Here's how the part is built. I have some questions about the finished solid (model axes, mm). Give positions to 0.01 mm unless a question says otherwise; leave off trailing zeros. Loops run counter-clockwise (first coordinate to the right, second up) from the corner with the lowest first, then second, coordinate; pieces in that order, holes last. Notation, with made-up numbers: (29.5, 76) - (60.5, 76) arc R14 ccw to (60.5, 99) - close; hole circle Ø4 at (34.5, -27.5). An arc over 180 degrees is marked (long way). Use a Markdown table: item, result.
from build123d import *

# Parameters (mm, degrees)
BOSS_EXTRUDE2_DEPTH = 0.2
BOSS_EXTRUDE3_DEPTH = 0.2


with BuildPart() as part:
    # Sketch1 → Revolve1 (revolve)
    with BuildSketch(Plane.XY):
        with BuildLine():
            Line((-1.375, 7.8), (1.375, 7.8))
            Line((1.375, 7.8), (1.375, 12.1))
            ThreePointArc((1.375, 12.1), (1.169974747, 12.594974747), (0.675, 12.8))
            Line((0.675, 12.8), (0.625, 12.8))
            Line((0.625, 12.8), (0.625, 13.6))
            ThreePointArc((0.625, 13.6), (0.478553391, 13.953553391), (0.125, 14.1))
            Line((0.125, 14.1), (-1.075, 14.1))
            ThreePointArc((-1.075, 14.1), (-1.287132034, 14.012132034), (-1.375, 13.8))
            Line((-1.375, 13.8), (-1.375, 7.8))
        make_face()
    revolve(axis=Axis((-11.93322357, 7.8, 0), (1, 0, 0)))

    # Sketch3 → Boss-Extrude2 (add)
    with BuildSketch(Plane(origin=(1.375, 0, 0), x_dir=(0, 0, -1), z_dir=(1, 0, 0))):
        Polygon((-2, 8), (-2, -1), (-1.25, -1), (-1.25, 0), (1.25, 0), (1.25, 8), align=None)
    extrude(amount=BOSS_EXTRUDE2_DEPTH)

    # Sketch5 → Boss-Extrude3 (add)
    with BuildSketch(Plane(origin=(-1.375, 0, -1.375), x_dir=(0, 0, -1), z_dir=(1, 0, 0))):
        Polygon((0.625, -1), (0.625, 8), (-2.625, 8), (-2.625, 0), (-0.125, 0), (-0.125, -1), align=None)
    extrude(amount=-BOSS_EXTRUDE3_DEPTH)


solid = part.part
(1) Suppose I cut it at C-C on y = 7.8. Write out the boundary of the cut face in (x, z) (3 decimals).
A:
| item | result |
|---|---|
| outline | (-1.575, -2) - (-1.375, -2) - (-1.375, -6) arc R0.3 ccw to (-1.075, -6.3) - (0.125, -6.3) arc R0.5 ccw to (0.625, -5.8) - (0.625, -5) - (0.675, -5) arc R0.7 ccw to (1.375, -4.3) - (1.375, -1.25) - (1.575, -1.25) - (1.575, 2) - (1.375, 2) - (1.375, 4.3) arc R0.7 ccw to (0.675, 5) - (0.625, 5) - (0.625, 5.8) arc R0.5 ccw to (0.125, 6.3) - (-1.075, 6.3) arc R0.3 ccw to (-1.375, 6) - (-1.375, 1.25) - (-1.575, 1.25) - close |
(2) Suppose I cut it at B-B on z = 0. Write out the boundary of the cut face in (x, y) (3 decimals), plus the area to 3 significant figures.
A:
| item | result |
|---|---|
| outline | (-1.575, 0) - (-1.375, 0) - (-1.375, 1.8) arc R0.3 ccw to (-1.075, 1.5) - (0.125, 1.5) arc R0.5 ccw to (0.625, 2) - (0.625, 2.8) - (0.675, 2.8) arc R0.7 ccw to (1.375, 3.5) - (1.375, 0) - (1.575, 0) - (1.575, 8) - (1.375, 8) - (1.375, 12.1) arc R0.7 ccw to (0.675, 12.8) - (0.625, 12.8) - (0.625, 13.6) arc R0.5 ccw to (0.125, 14.1) - (-1.075, 14.1) arc R0.3 ccw to (-1.375, 13.8) - (-1.375, 8) - (-1.575, 8) - close |
| area | 35.5 mm2 |
(3) Suppose I cut it at A-A on y = 1. Write out the boundary of the cut face in (x, z) (3 decimals).
A:
| item | result |
|---|---|
| outline | (-1.575, -2) - (-1.375, -2) - (-1.375, 1.25) - (-1.575, 1.25) - close; (1.375, -1.25) - (1.575, -1.25) - (1.575, 2) - (1.375, 2) - close |
(4) We'd pull the mould along X, two halves only. Please class faces 1 (the face through (-1.375, 1, 0)), 2 (the face through (-1.575, 4, 0)), 3 (the face through (1.575, 4, 0)): pulls with the +X half, pulls with the -X half, needs draft (parallel to the pull), parting line crosses it, or undercut.
A:
| item | result |
|---|---|
| face 1 | undercut |
| face 2 | pulls with the -X half |
| face 3 | pulls with the +X half |
(5) Will this pin go through, and if not, where does the flat tip stop? pin 1 (2 mm diameter, centred on y = 5.5, z = 4, fed in from -X) (3 decimals).
A:
| item | result |
|---|---|
| pin 1 | x = -1.375 |
(6) If I drill on line 1 (X direction, y = 5.75, z = 3) (3 decimals); line 2 (X direction, y = 5.5, z = -4.5) (3 decimals); line 3 (Z direction, x = 1.45, y = 5.75), over which ranges is the centre line in solid material (lowest first)?
A:
| item | result |
|---|---|
| line 1 | -1.375 to 1.375 |
| line 2 | -1.375 to 0.625 |
| line 3 | -1.25 to 2 |
(7) Suppose I cut it at D-D on x = -0.5. Write out the boundary of the cut face in (y, z), plus the area to 3 significant figures.
A:
| item | result |
|---|---|
| outline | circle Ø12.6 at (7.8, 0) |
| area | 125 mm2 |
